Read the model definition and answer for the solid it produces. Units are mm, in the model's axes. A direction names the side the tool comes from. Coordinates: 2 decimals unless noted, no trailing zeros. Write each loop counter-clockwise with the first axis right and the second up, starting at its lowest first coordinate (ties: lowest second). Pieces come first, ordered by that corner, then holes.
(1) The part is cut by section D-D, the plane x = -4. Determine the outline of the cut face in (y, z).
(2) Determine the mould class of faces 4 (the cylindrical face through (20.843, 3.042, 0.72)), 5 (the flat face through (18.128, 3, -12)), 6 (the cylindrical face through (-19.571, 3.042, 0.736)) for opening direction X: pulls with the +X half, pulls with the -X half, needs draft (parallel to the pull), parting line crosses it, or undercut.
(3) Straight lines are drawn through the part: line 1 along X through (y, z) = (2.8, -20.5); line 2 along X through (y, z) = (1, -3.75); line 3 along X through (y, z) = (2.05, -19.5). For each, find the intervals that lie inside material, in ascending order.
(4) The part is cut by section C-C, the plane y = 0.75. Determine the outline of the cut face in (x, z).
(5) Which of the six approach directions +Z, -Z, +X, -X, +Y, -Y give full straight-line access (tool end or side, diameter ignored) to faces 1 (the flat face through (-19.872, 3, -9)), 2 (the flat face through (-16.872, 3, -12)), 3 (the flat face through (26, 3, -18.979))?
(6) The part is cut by section B-B, the plane z = -9. Determine the outline of the cut face in (x, y).
(7) The part is cut by section A-A, the plane y = 3. Determine the outline of the cut face in (x, z).
(8) Given pin 1 (3 mm diameter, centred on y = 4, z = -10.5, fed in from +X); pin 2 (1.8 mm diameter, centred on x = -22.87, y = 3, fed in from +Z); pin 3 (3 mm diameter, centred on x = 17.5, y = 5, fed in from -Z); pin 4 (1.8 mm diameter, centred on x = 5, y = 2, fed in from -Z), each flat-ended and moving along its own axis, determine where each tip first touches the part or whether it passes through.
```python
from build123d import *

# Parameters (mm, degrees)
SKETCH1_W           = 6
SKETCH1_H           = 3
SKETCH1_W_2         = 41
BOSS_EXTRUDE1_DEPTH = 6
SKETCH2_R           = 1.5
CUT_EXTRUDE1_DEPTH  = 6
FILLET1_R           = 1
FILLET2_R           = 1
FILLET3_R           = 1
FILLET4_R           = 1


with BuildPart() as part:
    # Sketch1 → Boss-Extrude1 (new body)
    with BuildSketch(Plane(origin=(0, 0, 0), x_dir=(1, 0, 0), z_dir=(0, 1, 0))):
        with Locations((-22.87164751, 20.478927203)):
            Rectangle(SKETCH1_W, SKETCH1_H)
        Polygon((-19.87164751, 18.978927203), (-19.87164751, 1.978927203), (-16.87164751, 1.978927203), (-16.87164751, 21.978927203), (-19.87164751, 21.978927203), align=None)
        with Locations((0.62835249, 0.478927203)):
            Rectangle(SKETCH1_W_2, SKETCH1_H)
        Polygon((18.12835249, 21.978927203), (18.12835249, 1.978927203), (21.12835249, 1.978927203), (21.12835249, 18.978927203), (21.12835249, 21.978927203), align=None)
        with Locations((24.12835249, 20.478927203)):
            Rectangle(SKETCH1_W, SKETCH1_H)
    extrude(amount=BOSS_EXTRUDE1_DEPTH)

    # Sketch2 → Cut-Extrude1 (cut)
    with BuildSketch(Plane.XY.offset(-18.978927203)):
        with Locations((-22.87164751, 3)):
            Circle(SKETCH2_R)
        with Locations((24.12835249, 3)):
            Circle(SKETCH2_R)
    extrude(amount=-CUT_EXTRUDE1_DEPTH, mode=Mode.SUBTRACT)

    # Fillet1
    fillet1_edges = [part.edges().sort_by_distance(p)[0] for p in [
        (-19.87164751, 3, -18.978927203),
    ]]
    fillet(fillet1_edges, radius=FILLET1_R)

    # Fillet2
    fillet2_edges = [part.edges().sort_by_distance(p)[0] for p in [
        (21.12835249, 3, -18.978927203),
    ]]
    fillet(fillet2_edges, radius=FILLET2_R)

    # Fillet3
    fillet3_edges = [part.edges().sort_by_distance(p)[0] for p in [
        (21.12835249, 3, 1.021072797),
    ]]
    fillet(fillet3_edges, radius=FILLET3_R)

    # Fillet4
    fillet4_edges = [part.edges().sort_by_distance(p)[0] for p in [
        (-19.87164751, 3, 1.021072797),
    ]]
    fillet(fillet4_edges, radius=FILLET4_R)


solid = part.part
```
Computed:
1. outline: (0, -1.98) - (6, -1.98) - (6, 1.02) - (0, 1.02) - close
2. face 4: pulls with the +X half
2. face 5: undercut
2. face 6: pulls with the -X half
3. line 1: x = -25.87 to -24.36, -21.39 to -16.87, 18.13 to 22.64, 25.61 to 27.13
3. line 2: x = -19.87 to -16.87, 18.13 to 21.13
3. line 3: x = -25.87 to -24.03, -21.71 to -16.87, 18.13 to 22.97, 25.29 to 27.13
4. outline: (-25.87, -21.98) - (-16.87, -21.98) - (-16.87, -1.98) - (18.13, -1.98) - (18.13, -21.98) - (27.13, -21.98) - (27.13, -18.98) - (22.13, -18.98) arc R1 cw to (21.13, -17.98) - (21.13, 0.02) arc R1 ccw to (20.13, 1.02) - (-18.87, 1.02) arc R1 ccw to (-19.87, 0.02) - (-19.87, -17.98) arc R1 cw to (-20.87, -18.98) - (-25.87, -18.98) - close
5. face 1: +Z, -X, +Y, -Y
5. face 2: -Z, +Y, -Y
5. face 3: +Z, +X, +Y, -Y
6. outline: (-19.87, 0) - (-16.87, 0) - (-16.87, 6) - (-19.87, 6) - close; (18.13, 0) - (21.13, 0) - (21.13, 6) - (18.13, 6) - close
7. outline: (-25.87, -21.98) - (-24.37, -21.98) - (-24.37, -18.98) - (-25.87, -18.98) - close; (-21.37, -21.98) - (-16.87, -21.98) - (-16.87, -1.98) - (18.13, -1.98) - (18.13, -21.98) - (22.63, -21.98) - (22.63, -18.98) - (22.13, -18.98) arc R1 cw to (21.13, -17.98) - (21.13, 0.02) arc R1 ccw to (20.13, 1.02) - (-18.87, 1.02) arc R1 ccw to (-19.87, 0.02) - (-19.87, -17.98) arc R1 cw to (-20.87, -18.98) - (-21.37, -18.98) - close; (25.63, -21.98) - (27.13, -21.98) - (27.13, -18.98) - (25.63, -18.98) - close
8. pin 1: stops at x = 21.13
8. pin 2: passes through
8. pin 3: stops at z = -21.98
8. pin 4: stops at z = -1.98
